Read the model definition and answer for the solid it produces. Units are mm, in the model's axes. Face numbers are marked on the shaded views. A direction names the side the tool comes from. Coordinates: 2 decimals unless noted, no trailing zeros. Order: outer loops, then holes, each group sorted by start corner. A loop starts at its lowest first (then second) coordinate and runs counter-clockwise, first axis right, second up. Notation, with made-up numbers: (5, 19.5) - (53, 19.5) arc R16 ccw to (53, 42.5) - close; hole circle Ø8 at (50.25, 8). An arc over 180 degrees is marked (long way). Use one line per item in the form item = value. Start each with the question number.
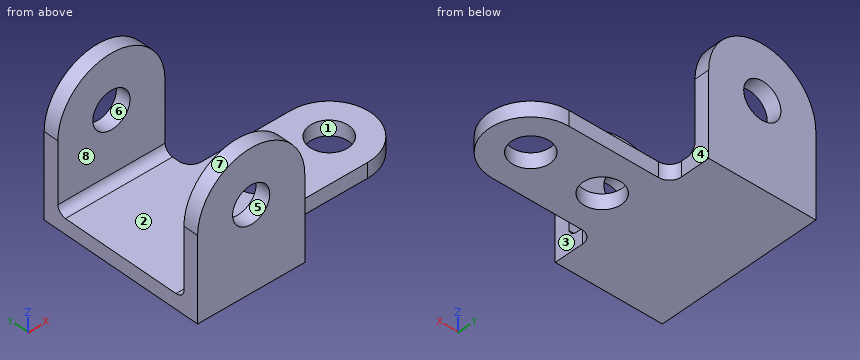
from build123d import *

# Parameters (mm, degrees)
F1_DEPTH = 7.9375
F2_W     = 57.15
F2_H     = 7.9375
F3_DEPTH = 76.2
F4_R     = 9.92251
F5_DEPTH = 88.901
F6_R     = 10.3251
F7_DEPTH = 25.4
F9_DEPTH = 57.15


with BuildPart() as f1:
    # F0 (on Top) → F1 (new body)
    with BuildSketch(Plane.XY):
        with BuildLine():
            Line((-9.525, -22.225), (38.1, -22.225))
            ThreePointArc((38.1, -22.225), (60.325, 0), (38.1, 22.225))
            Line((38.1, 22.225), (-9.525, 22.225))
            ThreePointArc((-9.525, 22.225), (-14.015128, 24.084872), (-15.875, 28.575))
            Line((-15.875, 28.575), (-15.875, 44.45))
            Line((-15.875, 44.45), (-73.025, 44.45))
            Line((-73.025, 44.45), (-73.025, -44.45))
            Line((-73.025, -44.45), (-15.875, -44.45))
            Line((-15.875, -44.45), (-15.875, -28.575))
            ThreePointArc((-15.875, -28.575), (-14.015128, -24.084872), (-9.525, -22.225))
        make_face()
    extrude(amount=F1_DEPTH)

    # F2 (on face) → F3 (join)
    with BuildSketch(Plane.XY.offset(7.9375)):
        with Locations((-44.45, 40.48125)):
            Rectangle(F2_W, F2_H)
        with Locations((-44.45, -40.48125)):
            Rectangle(F2_W, F2_H)
    extrude(amount=F3_DEPTH)

    # F4 (on face) → F5 (cut, through all)
    with BuildSketch(Plane.XZ.offset(44.45)):
        with BuildLine():
            ThreePointArc((-73.025, 44.45), (-44.45, 73.025), (-15.875, 44.45))
            Line((-15.875, 44.45), (-15.875, 84.1375))
            Line((-15.875, 84.1375), (-73.025, 84.1375))
            Line((-73.025, 84.1375), (-73.025, 44.45))
        make_face()
        with Locations((-44.45, 44.45)):
            Circle(F4_R)
    extrude(amount=-F5_DEPTH, mode=Mode.SUBTRACT)

    # F6 (on face) → F7 (cut)
    with BuildSketch(Plane.XY.offset(7.9375)):
        with Locations((38.1, 0)):
            Circle(F6_R)
        Circle(F6_R)
    extrude(amount=-F7_DEPTH, mode=Mode.SUBTRACT)

    # F8 (on face) → F9 (join)
    with BuildSketch(Plane(origin=(-73.025, 0, 0), x_dir=(0, -1, 0), z_dir=(-1, 0, 0))):
        with BuildLine():
            Line((-36.5125, 12.286079), (-36.5125, 13.082203))
            ThreePointArc((-36.5125, 13.082203), (-36.529165, 12.684141), (-36.5125, 12.286079))
        make_face()
        with BuildLine():
            Line((-31.378329, 7.9375), (-32.155001, 7.9375))
            ThreePointArc((-32.155001, 7.9375), (-31.766665, 7.921641), (-31.378329, 7.9375))
        make_face()
        with BuildLine():
            ThreePointArc((-32.155001, 7.9375), (-35.130808, 9.313096), (-36.5125, 12.286079))
            Line((-36.5125, 12.286079), (-36.5125, 7.9375))
            Line((-36.5125, 7.9375), (-32.155001, 7.9375))
        make_face()
        with BuildLine():
            Line((36.5125, 14.030189), (36.5125, 11.369799))
            ThreePointArc((36.5125, 11.369799), (36.702037, 12.699994), (36.5125, 14.030189))
        make_face()
        with BuildLine():
            ThreePointArc((36.5125, 11.369799), (34.801446, 8.893304), (31.947121, 7.9375))
            Line((31.947121, 7.9375), (36.5125, 7.9375))
            Line((36.5125, 7.9375), (36.5125, 11.369799))
        make_face()
    extrude(amount=-F9_DEPTH)


solid = f1.part
Q1. A cutting plane is placed at C-C (y = 0). Give the vertices of the cut face in (x, z) (1 decimal).
Q2. Consider probe 1 along Y at (x, z) = (38, 3) (3 decimals); probe 2 along Y at (x, z) = (-33, 38); probe 3 along Z at (x, y) = (-23, 0.5). Determine where each line is inside the solid, lowest interval first.
Q3. For a pull along Z with two mould halves and no side action, classify the marked faces 6, 7 and 8 as +Z half, -Z half, draft (parallel to the pull), parting line (faces both ways), or undercut.
Q4. A cutting plane is placed at D-D (x = 0). Give the vertices of the cut face in (y, z) (1 decimal).
Q5. Given P1, Ø8.5, axis at x = 6, z = 5, coming from the +Y side (3 decimals); P2, Ø17.5, axis at y = 36.5, z = 25, coming from the +X side (3 decimals); P3, Ø8.5, axis at x = 21, z = 2.5, coming from the -Y side (3 decimals); P4, Ø3, axis at y = -7.5, z = 9, coming from the -X side (3 decimals), each flat-ended and moving along its own axis, determine where each tip first touches the part or whether it passes through.
Q6. A cutting plane is placed at B-B (x = -44.45). Give the number of separate pieces and of enclosed holes in the cut face, then the cut area to 3 significant figures.
Q7. Which of the six approach directions +Z, -Z, +X, -X, +Y, -Y give full straight-line access (tool end or side, diameter ignored) to the marked faces 1, 2, 3, 4 and 5?
Result sheet:
q1.outline = (-73, 0) - (-10.3, 0) - (-10.3, 7.9) - (-73, 7.9) - close; (10.3, 0) - (27.8, 0) - (27.8, 7.9) - (10.3, 7.9) - close; (48.4, 0) - (60.3, 0) - (60.3, 7.9) - (48.4, 7.9) - close
q2.probe_1 = -22.225 to -10.325, 10.325 to 22.225
q2.probe_2 = -44.45 to -36.51, 36.51 to 44.45
q2.probe_3 = 0 to 7.94
q3.face_6 = undercut
q3.face_7 = +Z half
q3.face_8 = draft
q4.outline = (-22.2, 0) - (-10.3, 0) - (-10.3, 7.9) - (-22.2, 7.9) - close; (10.3, 0) - (22.2, 0) - (22.2, 7.9) - (10.3, 7.9) - close
q5.P1 = 22.225
q5.P2 = -15.875
q5.P3 = -22.225
q5.P4 = -73.025
q6.separate_pieces = 3
q6.enclosed_holes = 0
q6.area = 1,430 mm^2
q7.face_1 = +Z, -Z
q7.face_2 = +Z, +X, -X
q7.face_3 = +Z, -Z, +X, -Y
q7.face_4 = +Z, -Z, +X, +Y
q7.face_5 = +Y, -Y
